Geometry check sheet. Reference: the model listing, model coordinates, mm. Face numbers are marked on the shaded views. Give positions to 0.01 mm unless a question says otherwise; leave off trailing zeros. Loops run counter-clockwise (first coordinate to the right, second up) from the corner with the lowest first, then second, coordinate; pieces in that order, holes last.
```python
from build123d import *

# Parameters (mm, degrees)
SKETCH1_W                  = 50
SKETCH1_H                  = 50
EXTRUDE1_DEPTH             = 5
LPATTERN1_COUNT            = 2
LPATTERN1_PITCH            = 40
LPATTERN1_COUNT_DIR2       = 2
LPATTERN1_PITCH_DIR2       = 40
F_1_1_DIAMETER_HOLE1_D     = 25.4
F_1_1_DIAMETER_HOLE1_DEPTH = 6
F_1_1_DIAMETER_HOLE1_TIP   = 7.630929862


with BuildPart() as part:
    # Sketch1 → Extrude1 (new body)
    with BuildSketch(Plane(origin=(0, 0, 0), x_dir=(1, 0, 0), z_dir=(0, 1, 0))):
        Rectangle(SKETCH1_W, SKETCH1_H)
    extrude(amount=EXTRUDE1_DEPTH)

    # Sketch2 → M3 Clearance Hole1 (revolve, cut)
    with BuildSketch(Plane(origin=(-20, 5, 20), x_dir=(0, 0, 1), z_dir=(1, 0, 0))):
        Polygon((0, 0), (0, 6.96137699), (1.6, 6), (1.6, 0), align=None)
    m3_clearance_hole1 = revolve(axis=Axis((-20, 11.35, 20), (0, -1, 0)), mode=Mode.SUBTRACT)

    # LPattern1: M3 Clearance Hole1 2 × 2
    with Locations(*[(j * LPATTERN1_PITCH_DIR2, 0, -i * LPATTERN1_PITCH) for i in range(LPATTERN1_COUNT) for j in range(LPATTERN1_COUNT_DIR2) if (i, j) != (0, 0)]):
        add(m3_clearance_hole1, mode=Mode.SUBTRACT)

    # 1 (1) Diameter Hole1
    with Locations(Plane.ZX.offset(5)):
        with Locations((0, 0)):
            Hole(F_1_1_DIAMETER_HOLE1_D / 2, depth=F_1_1_DIAMETER_HOLE1_DEPTH)
            with Locations((0, 0, -(F_1_1_DIAMETER_HOLE1_DEPTH + F_1_1_DIAMETER_HOLE1_TIP / 2))):  # 118° drill point
                Cone(0, F_1_1_DIAMETER_HOLE1_D / 2, F_1_1_DIAMETER_HOLE1_TIP, mode=Mode.SUBTRACT)


solid = part.part
```
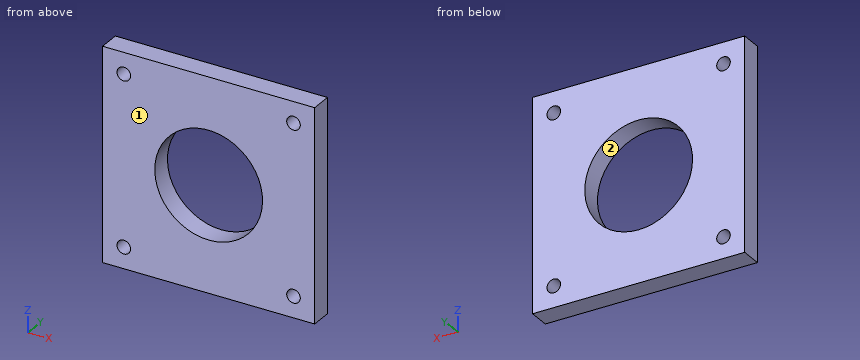
1) Sectioned sample at D-D on z = 0. Enter the section's corners in (x, y), plus the area to 3 significant figures.
2) Sectioned sample at C-C on x = -20. Enter the section's corners in (y, z).
3) Mould release check, pull along Z, two halves, no side actions. Record for the marked faces 1 and 2: +Z half, -Z half, draft (parallel to the pull), parting line (faces both ways), or undercut.
4) Sectioned sample at A-A on z = -20. Enter the section's corners in (x, y), plus the area to 3 significant figures.
5) Scan lines: line 1 along Z through (x, y) = (-20, 1.4); line 2 along X through (y, z) = (2.2, 0). Record each from-to range of solid material in increasing order.
6) Sectioned sample at B-B on x = 0. Enter the section's corners in (y, z), plus the area to 3 significant figures.
Determined:
1. outline: (-25, 0) - (-12.7, 0) - (-12.7, 5) - (-25, 5) - close; (12.7, 0) - (25, 0) - (25, 5) - (12.7, 5) - close
1. area: 123 mm2
2. outline: (0, -25) - (5, -25) - (5, -21.6) - (0, -21.6) - close; (0, -18.4) - (5, -18.4) - (5, 18.4) - (0, 18.4) - close; (0, 21.6) - (5, 21.6) - (5, 25) - (0, 25) - close
3. face 1: draft
3. face 2: undercut
4. outline: (-25, 0) - (-21.6, 0) - (-21.6, 5) - (-25, 5) - close; (-18.4, 0) - (18.4, 0) - (18.4, 5) - (-18.4, 5) - close; (21.6, 0) - (25, 0) - (25, 5) - (21.6, 5) - close
4. area: 218 mm2
5. line 1: z = -25 to -21.6, -18.4 to 18.4, 21.6 to 25
5. line 2: x = -25 to -12.7, 12.7 to 25
6. outline: (0, -25) - (5, -25) - (5, -12.7) - (0, -12.7) - close; (0, 12.7) - (5, 12.7) - (5, 25) - (0, 25) - close
6. area: 123 mm2
